Read the model definition and answer for the solid it produces. Units are mm, in the model's axes. A direction names the side the tool comes from. Coordinates: 2 decimals unless noted, no trailing zeros. Order: outer loops, then holes, each group sorted by start corner. A loop starts at its lowest first (then second) coordinate and runs counter-clockwise, first axis right, second up. Notation, with made-up numbers: (-16.5, 5) -> (0.5, 5) arc R13 cw to (0.5, 23) -> close; hole circle Ø5 at (-33, 21). An arc over 180 degrees is marked (long way). Return JSON: item names as keys, results as strings. Group by question number.
```python
from build123d import *

# Parameters (mm, degrees)
SKETCH1_W           = 12.5
SKETCH1_H           = 2.5
SKETCH1_W_2         = 2.5
SKETCH1_H_2         = 12.5
SKETCH1_W_3         = 9
SKETCH1_H_3         = 6
BOSS_EXTRUDE1_DEPTH = 3
FILLET1_R           = 2
SKETCH1_4_W         = 3
SKETCH1_4_H         = 7.491405235
BOSS_EXTRUDE2_DEPTH = 8.4
SKETCH2_R           = 2.4
BOSS_EXTRUDE3_DEPTH = 3
FILLET2_R           = 8
SKETCH1_7_R         = 1.25
CUT_EXTRUDE2_DEPTH  = 53.505324486


with BuildPart() as part:
    # Sketch1 → Boss-Extrude1 (new body)
    with BuildSketch(Plane(origin=(0, 0, 0), x_dir=(1, 0, 0), z_dir=(0, 1, 0))):
        Polygon((-14.041444449, -20.12144272), (-14.041444449, -12.630037485), (-38.561763486, -12.630037485), (-38.561763486, -34.630037485), (-1.270220731, -34.630037485), (-1.270220731, -12.630037485), (-4.270220731, -12.630037485), (-4.270220731, -20.12144272), align=None)
        with Locations((-10.520220731, -30.880037485)):
            Rectangle(SKETCH1_W, SKETCH1_H, mode=Mode.SUBTRACT)
        with Locations((-34.020220731, -25.190037485)):
            Rectangle(SKETCH1_W_2, SKETCH1_H_2, mode=Mode.SUBTRACT)
        with Locations((-24.475907507, -25.190037485)):
            Rectangle(SKETCH1_W_3, SKETCH1_H_3, mode=Mode.SUBTRACT)
    extrude(amount=BOSS_EXTRUDE1_DEPTH)

    # Fillet1
    fillet1_edges = [part.edges().sort_by_distance(p)[0] for p in [
        (-14.041444449, 1.5, 20.12144272),
        (-4.270220731, 1.5, 20.12144272),
        (-1.270220731, 1.5, 34.630037485),
        (-38.561763486, 1.5, 34.630037485),
        (-38.561763486, 1.5, 12.630037485),
    ]]
    fillet(fillet1_edges, radius=FILLET1_R)

    # Sketch1_4 → Boss-Extrude2 (add)
    with BuildSketch(Plane(origin=(0, 0, 0), x_dir=(1, 0, 0), z_dir=(0, 1, 0))):
        with Locations((-2.770220731, -16.375740103)):
            Rectangle(SKETCH1_4_W, SKETCH1_4_H)
        Polygon((-4.270220731, -29.630037485), (-4.270220731, -32.130037485), (-4.270220731, -34.630037485), (-1.270220731, -34.630037485), (-1.270220731, -20.12144272), (-4.270220731, -20.12144272), align=None)
    extrude(amount=-BOSS_EXTRUDE2_DEPTH)

    # Sketch2 → Boss-Extrude3 (add)
    with BuildSketch(Plane(origin=(-1.270220731, 0, 0), x_dir=(0, 0, -1), z_dir=(1, 0, 0))):
        with Locations(Location((-25.530037485, -6, 0), (0, 0, 270))):
            Circle(SKETCH2_R)
    extrude(amount=BOSS_EXTRUDE3_DEPTH)

    # Fillet2
    fillet2_edges = [part.edges().sort_by_distance(p)[0] for p in [
        (-2.770220731, -8.4, 12.630037485),
        (-2.770220731, -8.4, 34.630037485),
    ]]
    fillet(fillet2_edges, radius=FILLET2_R)

    # Sketch1_7 → Cut-Extrude2 (cut, through all)
    with BuildSketch(Plane(origin=(0, 0, 0), x_dir=(1, 0, 0), z_dir=(0, 1, 0))):
        with Locations(Location((-19.270220731, -32.130037485, 0), (0, 0, 270))):
            Circle(SKETCH1_7_R)
        with Locations(Location((-19.270220731, -15.130037485, 0), (0, 0, 270))):
            Circle(SKETCH1_7_R)
    extrude(amount=CUT_EXTRUDE2_DEPTH, mode=Mode.SUBTRACT)


solid = part.part
```
1. Straight lines are drawn through the part: L1, parallel to X at y = 0.75, z = 26.25; L2, parallel to Z at x = -26, y = 0.25; L3, parallel to X at y = 1.5, z = 32. For each, find the intervals that lie inside material, in ascending order.
2. Find section A-A on z = 16. Determine the outline of the cut face in (x, y), and give its area (3 significant figures).
3. Which of the six approach directions +Z, -Z, +X, -X, +Y, -Y give full straight-line access (tool end or side, diameter ignored) to faces 1 (the face through (-13.47, 1.52, 19.52)), 2 (the face through (-3, 1, 12.63)), 3 (the face through (-2.749, -5.994, 14.911)), 4 (the face through (0.21, -5.69, 23.15)), 5 (the face through (-11, 1, 29.63))?
4. Find section C-C on y = -6. Determine the outline of the cut face in (x, z), and give its area (3 significant figures).
5. For a pull along Z with two mould halves and no side action, classify faces 6 (the face through (-38.562, 1, 24)), 7 (the face through (-1.87, 1.52, 34.06)), 8 (the face through (-32.77, 1, 25)) as released by +Z, released by -Z, zero draft, split by the parting line, or undercut.
6. Find section D-D on y = 1.75. Determine the outline of the cut face in (x, z).
7. Given pin 1 (3.5 mm diameter, centred on y = 2, z = 27.5, fed in from +X); pin 2 (1.5 mm diameter, centred on x = -8, y = 1.5, fed in from -Z); pin 3 (1.5 mm diameter, centred on x = -12.5, y = 1, fed in from -Z) (3 decimals), each flat-ended and moving along its own axis, determine where each tip first touches the part or whether it passes through.
Result:
{
 "1": {"L1": "-38.56 to -35.27, -32.77 to -28.98, -19.98 to -1.27", "L2": "12.63 to 22.19, 28.19 to 34.63", "L3": "-38.56 to -20.51, -18.03 to -16.77, -4.27 to -1.27"},
 "2": {"outline": "(-38.56, 0) -> (-20.17, 0) -> (-20.17, 3) -> (-38.56, 3) -> close; (-18.37, 0) -> (-14.04, 0) -> (-14.04, 3) -> (-18.37, 3) -> close; (-4.27, -6.92) -> (-1.27, -6.92) -> (-1.27, 3) -> (-4.27, 3) -> close", "area": "97.9 mm^2"},
 "3": {"face 1": "-Z, +Y, -Y", "face 2": "-Z, +X, -X, +Y, -Y", "face 3": "-Z, +X, -X, -Y", "face 4": "+X", "face 5": "+Y, -Y"},
 "4": {"outline": "(-4.27, 14.92) -> (-1.27, 14.92) -> (-1.27, 23.13) -> (1.73, 23.13) -> (1.73, 27.93) -> (-1.27, 27.93) -> (-1.27, 32.34) -> (-4.27, 32.34) -> close", "area": "66.7 mm^2"},
 "5": {"face 6": "zero draft", "face 7": "released by +Z", "face 8": "undercut"},
 "6": {"outline": "(-38.56, 14.63) arc R2 ccw to (-36.56, 12.63) -> (-14.04, 12.63) -> (-14.04, 18.12) arc R2 cw to (-12.04, 20.12) -> (-6.27, 20.12) arc R2 cw to (-4.27, 18.12) -> (-4.27, 12.63) -> (-1.27, 12.63) -> (-1.27, 32.63) arc R2 ccw to (-3.27, 34.63) -> (-36.56, 34.63) arc R2 ccw to (-38.56, 32.63) -> close; hole (-35.27, 18.94) -> (-32.77, 18.94) -> (-32.77, 31.44) -> (-35.27, 31.44) -> close; hole (-28.98, 22.19) -> (-19.98, 22.19) -> (-19.98, 28.19) -> (-28.98, 28.19) -> close; hole circle Ø2.5 at (-19.27, 15.13); hole circle Ø2.5 at (-19.27, 32.13); hole (-16.77, 29.63) -> (-4.27, 29.63) -> (-4.27, 32.13) -> (-16.77, 32.13) -> close"},
 "7": {"pin 1": "x = -1.27", "pin 2": "z = 20.12", "pin 3": "z = 19.715"}
}
